Geometry check sheet. Reference: the model listing, model coordinates, mm. A direction names the side the tool comes from. Round coordinates to 2 decimals unless told otherwise and drop trailing zeros. Order: outer loops, then holes, each group sorted by start corner. A loop starts at its lowest first (then second) coordinate and runs counter-clockwise, first axis right, second up. Notation, with made-up numbers: (27, 47.25) - (45, 47.25) arc R26 ccw to (45, 68.25) - close; hole circle Ø2 at (9, 28). An arc over 180 degrees is marked (long way). Write each question's results on one line, items separated by ' | '.
```python
from build123d import *

# Parameters (mm, degrees)
BOSS_EXTRUDE2_DEPTH     = 2.54
BOSS_EXTRUDE3_DEPTH     = 18.288
FILLET1_R               = 2.54
SKETCH4_R               = 1.905
CUT_EXTRUDE1_DEPTH      = 26.4
CUT_EXTRUDE1_DEPTH_BACK = 1


with BuildPart() as part:
    # Sketch3 → Boss-Extrude2 (new body)
    with BuildSketch(Plane.XY):
        with BuildLine():
            Line((0, 82.55), (0, 0))
            Line((0, 0), (21.082, 0))
            Line((21.082, 0), (21.082, 29.480573053))
            ThreePointArc((21.082, 29.480573053), (7.366, 46.99), (21.082, 64.499426947))
            Line((21.082, 64.499426947), (21.082, 82.55))
            Line((21.082, 82.55), (0, 82.55))
        make_face()
    extrude(amount=BOSS_EXTRUDE2_DEPTH)

    # Sketch3<5> → Boss-Extrude3 (add)
    with BuildSketch(Plane.XY):
        with BuildLine():
            Line((21.082, 29.480573053), (21.082, 0))
            Line((21.082, 0), (25.4, 0))
            Line((25.4, 0), (25.4, 30.988))
            ThreePointArc((25.4, 30.988), (9.398, 46.99), (25.4, 62.992))
            Line((25.4, 62.992), (25.4, 82.55))
            Line((25.4, 82.55), (21.082, 82.55))
            Line((21.082, 82.55), (21.082, 64.499426947))
            ThreePointArc((21.082, 64.499426947), (7.366, 46.99), (21.082, 29.480573053))
        make_face()
    extrude(amount=BOSS_EXTRUDE3_DEPTH)

    # Fillet1
    fillet1_edges = [part.edges().sort_by_distance(p)[0] for p in [
        (21.082, 73.524713473, 2.54),
        (21.082, 14.740286527, 2.54),
        (7.366, 46.99, 2.54),
    ]]
    fillet(fillet1_edges, radius=FILLET1_R)

    # Sketch4 → Cut-Extrude1 (cut, two sides)
    with BuildSketch(Plane(origin=(0, 0, 0), x_dir=(0, 0, -1), z_dir=(1, 0, 0))) as cut_extrude1_sk:
        with Locations((-11.684, 14.740286527)):
            Circle(SKETCH4_R)
        with Locations((-11.684, 73.524713473)):
            Circle(SKETCH4_R)
    extrude(amount=CUT_EXTRUDE1_DEPTH, mode=Mode.SUBTRACT)
    extrude(cut_extrude1_sk.sketch, amount=-CUT_EXTRUDE1_DEPTH_BACK, mode=Mode.SUBTRACT)


solid = part.part
```
(1) Section check B-B (z = 8.25). Record the cut outline in (x, y).
Answers follow:
outline: (21.08, 0) - (25.4, 0) - (25.4, 30.99) arc R16 cw to (25.4, 62.99) - (25.4, 82.55) - (21.08, 82.55) - (21.08, 64.5) arc R18.03 ccw to (21.08, 29.48) - close
(2) Access from +Z, -Z, +X, -X, +Y, -Y to the whole of each face (thin tool, end or side, straight path). Record for faces 5 (the face through (20, 74, 3)), 6 (the face through (20, 15, 3)), 7 (the face through (5, 42, 2.54)).
Answers follow:
face 5: +Z, -X, +Y | face 6: +Z, -X, -Y | face 7: +Z, -X
(3) Material ranges on line 1 (Y direction, x = 12.5, z = 17.25); line 2 (X direction, y = 17.5, z = 12.25); line 3 (Z direction, x = 7.25, y = 15), recorded low to high.
Answers follow:
line 1: 34.39 to 37.52, 56.46 to 59.59 | line 2: 21.08 to 25.4 | line 3: 0 to 2.54
(4) Section check A-A (y = 46.99). Record the cut outline in (x, z).
Answers follow:
outline: (0, 0) - (9.4, 0) - (9.4, 18.29) - (7.37, 18.29) - (7.37, 5.08) arc R2.54 cw to (4.83, 2.54) - (0, 2.54) - close
(5) Draft check along Z on faces 1 (the face through (23.211, 75.414, 11.932)), 2 (the face through (10, 42, 0)), 3 (the face through (0, 42, 1)), 4 (the face through (23.211, 13.05, 10.805)). Enter one of: released by +Z, released by -Z, zero draft, split by the parting line, or undercut.
Answers follow:
face 1: undercut | face 2: released by -Z | face 3: zero draft | face 4: undercut
(6) Section check C-C (y = 7). Record the cut outline in (x, z).
Answers follow:
outline: (0, 0) - (25.4, 0) - (25.4, 18.29) - (21.08, 18.29) - (21.08, 5.08) arc R2.54 cw to (18.54, 2.54) - (0, 2.54) - close
(7) Depth check by flat-ended pin: pin 1 Ø9.5 at (x, y) = (6.5, 22) entering from +Z; pin 2 Ø2 at (x, y) = (19, 27) entering from +Z; pin 3 Ø8 at (x, z) = (13.5, 10) entering from -Y. Enter the tip coordinate at first touch or a pass-through.
Answers follow:
pin 1: z = 2.54 | pin 2: z = 3 | pin 3: y = 30.78
